```python
from build123d import *

# Parameters (mm, degrees)
SKETCH1_R           = 39.6748
SKETCH1_R_2         = 38.1
BOSS_EXTRUDE1_DEPTH = 685.8
CUT_EXTRUDE2_DEPTH  = 101.6


with BuildPart() as part:
    # Sketch1 → Boss-Extrude1 (new body)
    with BuildSketch(Plane(origin=(0, 0, 0), x_dir=(0, 0, -1), z_dir=(1, 0, 0))):
        Circle(SKETCH1_R)
        Circle(SKETCH1_R_2, mode=Mode.SUBTRACT)
    extrude(amount=BOSS_EXTRUDE1_DEPTH)

    # Sketch2 → Cut-Extrude2 (cut)
    with BuildSketch(Plane.ZY.offset(-50.8)):
        with BuildLine():
            Line((-1.5875, 39.643027114), (-1.5875, 38.066912716))
            ThreePointArc((-1.5875, 38.066912716), (0, 38.1), (1.5875, 38.066912716))
            Line((1.5875, 38.066912716), (1.5875, 39.643027114))
            ThreePointArc((1.5875, 39.643027114), (0, 39.6748), (-1.5875, 39.643027114))
        make_face()
        with BuildLine():
            Line((35.125618564, -18.446698229), (33.760663456, -17.65864103))
            ThreePointArc((33.760663456, -17.65864103), (32.995567884, -19.05), (32.173163456, -20.408271687))
            Line((32.173163456, -20.408271687), (33.538118564, -21.196328886))
            ThreePointArc((33.538118564, -21.196328886), (34.35938469, -19.8374), (35.125618564, -18.446698229))
        make_face()
        with BuildLine():
            Line((-33.538118564, -21.196328886), (-32.173163456, -20.408271687))
            ThreePointArc((-32.173163456, -20.408271687), (-32.995567884, -19.05), (-33.760663456, -17.65864103))
            Line((-33.760663456, -17.65864103), (-35.125618564, -18.446698229))
            ThreePointArc((-35.125618564, -18.446698229), (-34.35938469, -19.8374), (-33.538118564, -21.196328886))
        make_face()
    extrude(amount=-CUT_EXTRUDE2_DEPTH, mode=Mode.SUBTRACT)


solid = part.part
```
Verification items for the finished model (mm, model axes). Coordinates: 2 decimals unless noted, no trailing zeros. Order: outer loops, then holes, each group sorted by start corner. A loop starts at its lowest first (then second) coordinate and runs counter-clockwise, first axis right, second up. Notation, with made-up numbers: (-0.5, 60) -> (20.5, 60) arc R23 ccw to (20.5, 85) -> close; hole circle Ø4 at (70, -21). An arc over 180 degrees is marked (long way). Answer as CSV lines item,"result". Start each with the question number.
1) Release check for a two-part mould opening along Z. For faces 1 (the face through (338.099, -23.183, 30.235)), 2 (the face through (338.099, 26.814, 29.242)), 3 (the face through (685.8, 35.5, 14.9)) record: released by +Z, released by -Z, zero draft, split by the parting line, or undercut.
2) Gauge pin test, flat ends, axial feed: pin 1 Ø10 at (x, y) = (427.5, -28.5) entering from +Z; pin 2 Ø1.5 at (x, z) = (131.5, -16) entering from +Y; pin 3 Ø4 at (x, z) = (419.5, -28.5) entering from -Y. Record the tip position at first contact, or that the pin passes through.
3) Cross-section at C-C, the plane x = 458. Record the boundary of the cut face in (y, z).
4) Cross-section at B-B, the plane z = 14. Record the boundary of the cut face in (x, y), then the cut area to 3 significant figures.
5) Cross-section at A-A, the plane y = 0. Record the boundary of the cut face in (x, z).
6) Material ranges on L1, parallel to Y at x = 37.5, z = -0.5; L2, parallel to Y at x = 438, z = -3; L3, parallel to Z at x = 95.5, y = 29.5, recorded low to high. Write a range as [from, to].
Conclusion:
1,face 1,"undercut"
1,face 2,"split by the parting line"
1,face 3,"zero draft"
2,pin 1,"stops at z = 31.97"
2,pin 2,"stops at y = 36.63"
2,pin 3,"stops at y = -29.53"
3,outline,"circle Ø79.35 at (0, 0); hole circle Ø76.2 at (0, 0)"
4,outline,"(0, -37.12) -> (685.8, -37.12) -> (685.8, -35.43) -> (0, -35.43) -> close; (0, 35.43) -> (685.8, 35.43) -> (685.8, 37.12) -> (0, 37.12) -> close"
4,area,"2,320 mm²"
5,outline,"(0, -39.67) -> (685.8, -39.67) -> (685.8, -38.1) -> (0, -38.1) -> close; (0, 38.1) -> (685.8, 38.1) -> (685.8, 39.67) -> (0, 39.67) -> close"
6,L1,"y = [-39.67, -38.1], [38.1, 39.67]"
6,L2,"y = [-39.56, -37.98], [37.98, 39.56]"
6,L3,"z = [-26.53, -24.11], [24.11, 26.53]"
